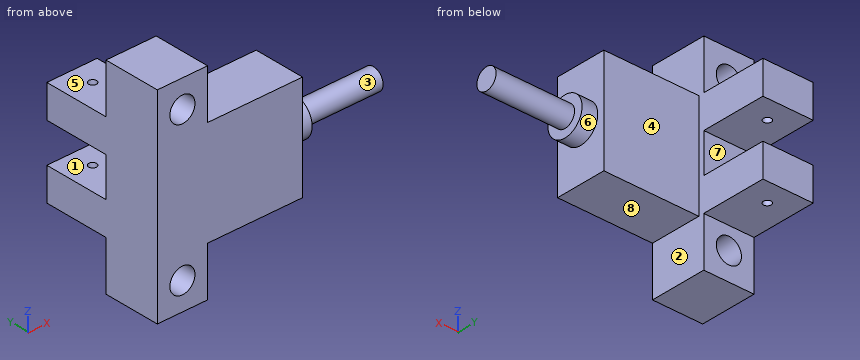
from build123d import *

# Parameters (mm, degrees)
AUFSATZ_LINEAR_AUSTRAGEN1_DEPTH = 26
SKIZZE2_W                       = 12.1
SKIZZE2_H                       = 6.3
SCHNITT_LINEAR_AUSTRAGEN1_DEPTH = 26
SKIZZE3_W                       = 6.4
SKIZZE3_H                       = 6.3
SCHNITT_LINEAR_AUSTRAGEN2_DEPTH = 8.3
SKIZZE4_W                       = 6.4
SKIZZE4_H                       = 5
SCHNITT_LINEAR_AUSTRAGEN3_DEPTH = 8.3
SKIZZE5_R                       = 0.5
SCHNITT_LINEAR_AUSTRAGEN4_DEPTH = 32.154293444
SKIZZE6_R                       = 1.6
SCHNITT_LINEAR_AUSTRAGEN5_DEPTH = 8.3
SKIZZE7_R                       = 2.4
AUFSATZ_LINEAR_AUSTRAGEN2_DEPTH = 2
SKIZZE8_R                       = 1.35
AUFSATZ_LINEAR_AUSTRAGEN3_DEPTH = 10


with BuildPart() as part:
    # Skizze1 → Aufsatz-Linear austragen1 (new body)
    with BuildSketch(Plane.XY):
        Polygon((0, 0), (0, 15.5), (6.4, 15.5), (6.4, 6.5), (18.5, 6.5), (18.5, 0), align=None)
    extrude(amount=AUFSATZ_LINEAR_AUSTRAGEN1_DEPTH)

    # Skizze2 → Schnitt-Linear austragen1 (cut)
    with BuildSketch(Plane(origin=(0, 6.5, 0), x_dir=(1, 0, 0), z_dir=(0, 1, 0))):
        with Locations((12.45, -22.85)):
            Rectangle(SKIZZE2_W, SKIZZE2_H)
        with Locations((12.45, -3.15)):
            Rectangle(SKIZZE2_W, SKIZZE2_H)
    extrude(amount=-SCHNITT_LINEAR_AUSTRAGEN1_DEPTH, mode=Mode.SUBTRACT)

    # Skizze3 → Schnitt-Linear austragen2 (cut)
    with BuildSketch(Plane(origin=(0, 15.5, 0), x_dir=(1, 0, 0), z_dir=(0, 1, 0))):
        with Locations((3.2, -22.85)):
            Rectangle(SKIZZE3_W, SKIZZE3_H)
        with Locations((3.2, -3.15)):
            Rectangle(SKIZZE3_W, SKIZZE3_H)
    extrude(amount=-SCHNITT_LINEAR_AUSTRAGEN2_DEPTH, mode=Mode.SUBTRACT)

    # Skizze4 → Schnitt-Linear austragen3 (cut)
    with BuildSketch(Plane(origin=(0, 15.5, 0), x_dir=(1, 0, 0), z_dir=(0, 1, 0))):
        with Locations((3.2, -13)):
            Rectangle(SKIZZE4_W, SKIZZE4_H)
    extrude(amount=-SCHNITT_LINEAR_AUSTRAGEN3_DEPTH, mode=Mode.SUBTRACT)

    # Skizze5 → Schnitt-Linear austragen4 (cut, through all)
    with BuildSketch(Plane.XY.offset(19.7)):
        with Locations((3.2, 12.6)):
            Circle(SKIZZE5_R)
    extrude(amount=-SCHNITT_LINEAR_AUSTRAGEN4_DEPTH, mode=Mode.SUBTRACT)

    # Skizze6 → Schnitt-Linear austragen5 (cut)
    with BuildSketch(Plane(origin=(0, 7.2, 0), x_dir=(1, 0, 0), z_dir=(0, 1, 0))):
        with Locations(Location((3.2, -22.5, 0), (0, 0, 270))):
            Circle(SKIZZE6_R)
        with Locations(Location((3.2, -3.5, 0), (0, 0, 270))):
            Circle(SKIZZE6_R)
    extrude(amount=-SCHNITT_LINEAR_AUSTRAGEN5_DEPTH, mode=Mode.SUBTRACT)

    # Skizze7 → Aufsatz-Linear austragen2 (add)
    with BuildSketch(Plane(origin=(18.5, 0, 0), x_dir=(0, 0, -1), z_dir=(1, 0, 0))):
        with Locations(Location((-13, 3.25, 0), (0, 0, 180))):
            Circle(SKIZZE7_R)
    extrude(amount=AUFSATZ_LINEAR_AUSTRAGEN2_DEPTH)

    # Skizze8 → Aufsatz-Linear austragen3 (add)
    with BuildSketch(Plane(origin=(20.5, 0, 0), x_dir=(0, 0, -1), z_dir=(1, 0, 0))):
        with Locations((-13, 3.25)):
            Circle(SKIZZE8_R)
    extrude(amount=AUFSATZ_LINEAR_AUSTRAGEN3_DEPTH)


solid = part.part
Model file for the job. Use its own axes, mm. Face numbers are marked on the shaded views. A direction names the side the tool comes from. Give positions to 0.01 mm unless a question says otherwise; leave off trailing zeros. Order: outer loops, then holes, each group sorted by start corner. A loop starts at its lowest first (then second) coordinate and runs counter-clockwise, first axis right, second up. Notation, with made-up numbers: (59.5, 58) - (91.5, 58) arc R18 ccw to (91.5, 80) - close; hole circle Ø1 at (35, 40.5). An arc over 180 degrees is marked (long way). Write item = value, one per line. Start each with the question number.
1. Cut at C-C, the plane y = 9.75. List the corners of the cut face in (x, z), and give its area (3 significant figures).
2. Cut at D-D, the plane x = 3.2. List the corners of the cut face in (y, z), and give its area (3 significant figures).
3. Drop flat-ended pins along their axis: P1, Ø5, axis at x = 11.5, y = 3, coming from the -Z side; P2, Ø2.5, axis at x = 3.2, z = 3.5, coming from the -Y side; P3, Ø1.9, axis at x = 2, y = 11, coming from the +Z side; P4, Ø2, axis at x = 19, z = 12.5, coming from the +Y side. Give the stop position or say it passes through.
4. Probe line 1 along Y through (x, z) = (3.2, 17.45); line 2 along X through (y, z) = (3.75, 22.5); line 3 along Z through (x, y) = (1.5, 12.25). List the from-to ranges inside material, lowest first.
5. Two-plate mould, pull along Z, no slides. Class the marked faces 1, 2 and 3: pulls with the +Z half, pulls with the -Z half, needs draft (parallel to the pull), parting line crosses it, or undercut.
6. Which spindle directions (+Z, -Z, +X, -X, +Y, -Y) get a long thin tool onto all of the face, cutting with end or side? Do the marked faces 4, 5, 6, 7 and 8. Say none if no direction does.
7. Cut at B-B, the plane z = 3.5. List the corners of the cut face in (x, y).
8. Cut at A-A, the plane y = 12.6. List the corners of the cut face in (x, z), and give its area (3 significant figures).
Taken from the geometry:
q1.outline = (0, 6.3) - (6.4, 6.3) - (6.4, 10.5) - (0, 10.5) - close; (0, 15.5) - (6.4, 15.5) - (6.4, 19.7) - (0, 19.7) - close
q1.area = 53.8 mm²
q2.outline = (0, 0) - (7.2, 0) - (7.2, 1.9) - (0, 1.9) - close; (0, 5.1) - (7.2, 5.1) - (7.2, 6.3) - (12.1, 6.3) - (12.1, 10.5) - (7.2, 10.5) - (7.2, 15.5) - (12.1, 15.5) - (12.1, 19.7) - (7.2, 19.7) - (7.2, 20.9) - (0, 20.9) - close; (0, 24.1) - (7.2, 24.1) - (7.2, 26) - (0, 26) - close; (13.1, 6.3) - (15.5, 6.3) - (15.5, 10.5) - (13.1, 10.5) - close; (13.1, 15.5) - (15.5, 15.5) - (15.5, 19.7) - (13.1, 19.7) - close
q2.area = 202 mm²
q3.P1 = 6.3
q3.P2 = through
q3.P3 = 19.7
q3.P4 = 6.5
q4.line_1 = 0 to 12.1, 13.1 to 15.5
q4.line_2 = 0 to 1.6, 4.8 to 6.4
q4.line_3 = 6.3 to 10.5, 15.5 to 19.7
q5.face_1 = undercut
q5.face_2 = needs draft
q5.face_3 = parting line crosses it
q6.face_4 = +Z, -Z, +X, +Y
q6.face_5 = +Z, +X, -X, +Y
q6.face_6 = +X
q6.face_7 = +X, -X, +Y
q6.face_8 = -Z, +X, +Y, -Y
q7.outline = (0, 0) - (1.6, 0) - (1.6, 7.2) - (0, 7.2) - close; (4.8, 0) - (6.4, 0) - (6.4, 7.2) - (4.8, 7.2) - close
q8.outline = (0, 6.3) - (2.7, 6.3) - (2.7, 10.5) - (0, 10.5) - close; (0, 15.5) - (2.7, 15.5) - (2.7, 19.7) - (0, 19.7) - close; (3.7, 6.3) - (6.4, 6.3) - (6.4, 10.5) - (3.7, 10.5) - close; (3.7, 15.5) - (6.4, 15.5) - (6.4, 19.7) - (3.7, 19.7) - close
q8.area = 45.4 mm²
